Check sheet for the modelled part. Datum: model origin and axes. Units: mm. A direction names the side the tool comes from. Round coordinates to 2 decimals unless told otherwise and drop trailing zeros. Write each loop counter-clockwise with the first axis right and the second up, starting at its lowest first coordinate (ties: lowest second). Pieces come first, ordered by that corner, then holes.
from build123d import *

# Parameters (mm, degrees)
EXTRUDE_180_DEPTH      = 8
EXTRUDE_START          = 8
SKETCH_2_W             = 6
SKETCH_2_H             = 4
EXTRUDE_456_DEPTH      = 36
EXTRUDE_START_2        = 44
EXTRUDE_180_2_DEPTH    = 3
SKETCH_4_R             = 20
SKETCH_4_R_2           = 4
EXTRUDE_691_DEPTH      = 3
EXTRUDE_744_DEPTH      = 3
SKETCH_6_W             = 10
SKETCH_6_H             = 96
EXTRUDE_1_DEPTH        = 3
EXTRUDE_Y_1_DEPTH      = 3
SKETCH_8_W             = 10
SKETCH_8_H             = 96
EXTRUDE_1_2_DEPTH      = 3
EXTRUDE_Y_1_2_DEPTH    = 3
CUT_EXTRUDE_START      = 44
CUT_EXTRUDE_1136_DEPTH = 3
EXTRUDE_1227_DEPTH     = 3
SKETCH_12_R            = 5
EXTRUDE_1296_DEPTH     = 8
SKETCH_13_R            = 1.6
CUT_EXTRUDE_1367_DEPTH = 3
SKETCH_14_R            = 1.6
CUT_EXTRUDE_1428_DEPTH = 8
SKETCH_15_W            = 600
SKETCH_15_H            = 600
CUT_EXTRUDE_1488_DEPTH = 44
F_2MM_START            = 44
F_2MM_DEPTH            = 3
SKETCH_17_R            = 5
EXTRUDE_M3_DEPTH       = 3
SKETCH_18_R            = 5
EXTRUDE_3_DEPTH        = 3
SKETCH_19_R            = 5
EXTRUDE_4_DEPTH        = 3
SKETCH_20_R            = 1.6
CUT_EXTRUDE_M3_DEPTH   = 3
R7P8_75_R              = 7.8
R3P9_R                 = 3.9
F_2MM_45_47_START      = 44
SKETCH_21_W            = 600
SKETCH_21_H            = 600
F_2MM_45_47_DEPTH      = 1
FILLET_1_R             = 1.4
CHAMFER_1_SIZE         = 5
CHAMFER_1_SIZE_2       = 4.246045496
CHAMFER_1_SIZE_3       = 3.817956769
CHAMFER_1_SIZE_4       = 4.370160244
CHAMFER_1_SIZE_5       = 3.876090347
CHAMFER_1_SIZE_6       = 9.033398393


with BuildPart() as part:
    # 草图1 → Extrude 180 (new body)
    with BuildSketch(Plane.XY):
        Polygon((0, -115), (35.536954353, -109.371499374), (70.801069662, -90.621236665), (96.447115314, -62.633489027), (111.081470023, -29.764190187), (115, 0), (111.081470023, 29.764190187), (96.447115314, 62.633489027), (70.801069662, 90.621236665), (35.536954353, 109.371499374), (0, 115), (0, 111), (34.300886376, 105.567273309), (68.338423761, 87.46919365), (93.092433042, 60.454932887), (107.217766718, 28.728914006), (111, 0), (107.217766718, -28.728914006), (93.092433042, -60.454932887), (68.338423761, -87.46919365), (34.300886376, -105.567273309), (0, -111), align=None)
    extrude(amount=EXTRUDE_180_DEPTH)

    # 草图2 → Extrude 456 (add)
    with BuildSketch(Plane.XY.offset(EXTRUDE_START)):
        Polygon((35.584965419, -103.047126287), (37.439067386, -108.753465385), (33.634841321, -109.989533363), (31.780739354, -104.283194265), align=None)
        with Locations((112, 0)):
            Rectangle(SKETCH_2_W, SKETCH_2_H)
        Polygon((31.780739354, 104.283194265), (33.634841321, 109.989533363), (37.439067386, 108.753465385), (35.584965419, 103.047126287), align=None)
    extrude(amount=EXTRUDE_456_DEPTH)

    # 草图3 → Extrude 180 2 (add)
    with BuildSketch(Plane.XY.offset(EXTRUDE_START_2)):
        Polygon((0, -115), (35.536954353, -109.371499374), (70.801069662, -90.621236665), (96.447115314, -62.633489027), (111.081470023, -29.764190187), (115, 0), (111.081470023, 29.764190187), (96.447115314, 62.633489027), (70.801069662, 90.621236665), (35.536954353, 109.371499374), (0, 115), (0, 109), (33.682852387, 103.665160276), (67.10710081, 85.893172143), (91.415091906, 59.365654817), (105.285915066, 28.211275916), (109, 0), (105.285915066, -28.211275916), (91.415091906, -59.365654817), (67.10710081, -85.893172143), (33.682852387, -103.665160276), (0, -109), align=None)
    extrude(amount=EXTRUDE_180_2_DEPTH)



with BuildPart() as body_2:
    # 草图4 → Extrude 691 (new body)
    with BuildSketch(Plane.XY.offset(EXTRUDE_START_2)):
        Circle(SKETCH_4_R)
        Circle(SKETCH_4_R_2, mode=Mode.SUBTRACT)
    extrude(amount=EXTRUDE_691_DEPTH)


with BuildPart() as part_1:
    add(part.part)

    add(body_2.part)  # Extrude 744 merges body 2
    # 草图5 → Extrude 744 (add)
    with BuildSketch(Plane.XY.offset(EXTRUDE_START_2)):
        Polygon((17, -9), (113, -2.5), (113, 2.5), (17, 9), align=None)
    extrude(amount=EXTRUDE_744_DEPTH)

    # 草图6 → Extrude 1 (add)
    with BuildSketch(Plane.XY.offset(EXTRUDE_START_2)):
        with Locations((0, -64)):
            Rectangle(SKETCH_6_W, SKETCH_6_H)
    extrude(amount=EXTRUDE_1_DEPTH)

    # 草图7 → Extrude Y__-1 (add)
    with BuildSketch(Plane.XY.offset(EXTRUDE_START_2)):
        Polygon((60.213265383, 1.279918343), (91.234949037, -66.240061243), (87.165050963, -68.159938757), (54.786734617, -1.279918343), align=None)
    extrude(amount=EXTRUDE_Y_1_DEPTH)

    # 草图8 → Extrude 1 2 (add)
    with BuildSketch(Plane.XY.offset(EXTRUDE_START_2)):
        with Locations((0, 64)):
            Rectangle(SKETCH_8_W, SKETCH_8_H)
    extrude(amount=EXTRUDE_1_2_DEPTH)

    # 草图9 → Extrude Y__1 2 (add)
    with BuildSketch(Plane.XY.offset(EXTRUDE_START_2)):
        Polygon((54.786734617, 1.279918343), (87.165050963, 68.159938757), (91.234949037, 66.240061243), (60.213265383, -1.279918343), align=None)
    extrude(amount=EXTRUDE_Y_1_2_DEPTH)

    # 草图10 → Cut-Extrude 1136 (cut)
    with BuildSketch(Plane.XY.offset(CUT_EXTRUDE_START)):
        Polygon((18, -4.5), (18, 4.5), (80.33, 0), align=None)
    extrude(amount=CUT_EXTRUDE_1136_DEPTH, mode=Mode.SUBTRACT)

    # 草图11 → Extrude 1227 (add)
    with BuildSketch(Plane.XY.offset(EXTRUDE_START_2)):
        Polygon((-5, -107), (5, -107), (5, -116.208077798), (0, -117), (-3, -115), (-5, -112), align=None)
        Polygon((-5, 107), (5, 107), (5, 116.208077798), (0, 117), (-3, 115), (-5, 112), align=None)
    extrude(amount=EXTRUDE_1227_DEPTH)

    # 草图12 → Extrude 1296 (add)
    with BuildSketch(Plane.XY):
        with Locations((0, 112)):
            Circle(SKETCH_12_R)
        with Locations((0, -112)):
            Circle(SKETCH_12_R)
    extrude(amount=EXTRUDE_1296_DEPTH)

    # 草图13 → Cut-Extrude 1367 (cut)
    with BuildSketch(Plane.XY.offset(CUT_EXTRUDE_START)):
        with Locations((0, 112)):
            Circle(SKETCH_13_R)
        with Locations((0, -112)):
            Circle(SKETCH_13_R)
        with Locations((-6.717514421, -6.717514421)):
            Circle(SKETCH_13_R)
        with Locations((-6.717514421, 6.717514421)):
            Circle(SKETCH_13_R)
        with Locations((6.717514421, -6.717514421)):
            Circle(SKETCH_13_R)
        with Locations((6.717514421, 6.717514421)):
            Circle(SKETCH_13_R)
    extrude(amount=CUT_EXTRUDE_1367_DEPTH, mode=Mode.SUBTRACT)

    # 草图14 → Cut-Extrude 1428 (cut)
    with BuildSketch(Plane.XY):
        with Locations((0, 112)):
            Circle(SKETCH_14_R)
        with Locations((0, -112)):
            Circle(SKETCH_14_R)
    extrude(amount=CUT_EXTRUDE_1428_DEPTH, mode=Mode.SUBTRACT)

    # 草图15 → Cut-Extrude 1488 (cut)
    with BuildSketch(Plane.XY):
        Rectangle(SKETCH_15_W, SKETCH_15_H)
    extrude(amount=CUT_EXTRUDE_1488_DEPTH, mode=Mode.SUBTRACT)

    # 草图16 → 外圈径向加厚2mm (add)
    with BuildSketch(Plane.XY.offset(F_2MM_START)):
        Polygon((0, -117), (36.154988342, -111.273612407), (72.032392613, -92.197258172), (98.12445645, -63.722767097), (113.013321676, -30.281828277), (117, 0), (113.013321676, 30.281828277), (98.12445645, 63.722767097), (72.032392613, 92.197258172), (36.154988342, 111.273612407), (0, 117), (0, 114), (35.227937359, 108.420442858), (70.185408187, 89.833225911), (95.608444746, 62.088849992), (110.115544197, 29.505371142), (114, 0), (110.115544197, -29.505371142), (95.608444746, -62.088849992), (70.185408187, -89.833225911), (35.227937359, -108.420442858), (0, -114), align=None)
    extrude(amount=F_2MM_DEPTH)

    # 草图17 → M3铝柱上定位耳 (add)
    with BuildSketch(Plane.XY.offset(EXTRUDE_START_2)):
        with Locations((35.227937359, -108.420442858)):
            Circle(SKETCH_17_R)
    extrude(amount=EXTRUDE_M3_DEPTH)

    # 草图18 → 凸台-拉伸3 (add)
    with BuildSketch(Plane.XY.offset(EXTRUDE_START_2)):
        with Locations((114, 0)):
            Circle(SKETCH_18_R)
    extrude(amount=EXTRUDE_3_DEPTH)

    # 草图19 → 凸台-拉伸4 (add)
    with BuildSketch(Plane.XY.offset(EXTRUDE_START_2)):
        with Locations((35.227937359, 108.420442858)):
            Circle(SKETCH_19_R)
    extrude(amount=EXTRUDE_4_DEPTH)

    # 草图20 → 三处M3上层固定孔 (cut)
    with BuildSketch(Plane.XY.offset(CUT_EXTRUDE_START)):
        with Locations((35.227937359, -108.420442858)):
            Circle(SKETCH_20_R)
        with Locations((114, 0)):
            Circle(SKETCH_20_R)
        with Locations((35.227937359, 108.420442858)):
            Circle(SKETCH_20_R)
    extrude(amount=CUT_EXTRUDE_M3_DEPTH, mode=Mode.SUBTRACT)

    # 外侧梁根部圆角_R7p8_参考75度桨保
    r7p8_75_edges = [part_1.edges().sort_by_distance(p)[0] for p in [
        (5, -19.364916731, 45.5),
        (-5, -19.364916731, 45.5),
        (-5, 19.364916731, 45.5),
        (5, 19.364916731, 45.5),
    ]]
    fillet(r7p8_75_edges, radius=R7P8_75_R)

    # 端耳外缘圆角_R3p9_轮廓内收
    r3p9_edges = [part_1.edges().sort_by_distance(p)[0] for p in [
        (-5, -112, 45.5),
        (-5, 112, 45.5),
        (-3, -115, 45.5),
        (0, -117, 45.5),
        (0, 117, 45.5),
        (-3, 115, 45.5),
    ]]
    fillet(r3p9_edges, radius=R3P9_R)

    # 草图21 → 统一2mm板厚_上层保留45至47 (cut)
    with BuildSketch(Plane.XY.offset(F_2MM_45_47_START)):
        Rectangle(SKETCH_21_W, SKETCH_21_H)
    extrude(amount=F_2MM_45_47_DEPTH, mode=Mode.SUBTRACT)

    # 圆角1
    fillet_1_edges = [part_1.edges().sort_by_distance(p)[0] for p in [
        (18, -4.5, 46),
        (80.33, 0, 46),
        (18, 4.5, 46),
    ]]
    fillet(fillet_1_edges, radius=FILLET_1_R)

    # 倒角1
    # the kernel refuses this chamfer: 9.033398393, 5, 4.370160244, 4.246045496, 3.876090347, 3.817956769 mm, written as the material it adds along each edge
    with BuildSketch(Plane(origin=(108.631931923, -2.795754609, 45), x_dir=(-0.10321619689960815, -0.9946589449140752, 0), z_dir=(0, 0, 1))) as chamfer_1_piece_1:
        Polygon((CHAMFER_1_SIZE * 0.999621916911, -CHAMFER_1_SIZE * 0.0274958766106), (CHAMFER_1_SIZE_2 * 0.17017326961, -CHAMFER_1_SIZE_2 * 0.985414155772), (0, 0), align=None)
    extrude(amount=2)
    with BuildSketch(Plane(origin=(108.631931923, 2.795754609, 47), x_dir=(-0.9995678495067102, 0.02939581998398161, 0), z_dir=(0, 0, -1))) as chamfer_1_piece_2:
        Polygon((CHAMFER_1_SIZE_2 * 0.999270274205, CHAMFER_1_SIZE_2 * 0.0381958005112), (CHAMFER_1_SIZE * 0.159614119931, CHAMFER_1_SIZE * 0.987179483538), (0, 0), align=None)
    extrude(amount=2)
    with BuildSketch(Plane(origin=(89.191460159, -61.792323046, 45), x_dir=(0.6956068650639778, 0.7184226397294735, 0), z_dir=(0, 0, 1))) as chamfer_1_piece_3:
        Polygon((CHAMFER_1_SIZE * 0.999621916911, CHAMFER_1_SIZE * 0.0274958766106), (CHAMFER_1_SIZE_3 * 0.36240953925, CHAMFER_1_SIZE_3 * 0.932018951466), (0, 0), align=None)
    extrude(amount=2)
    with BuildSketch(Plane(origin=(89.191460159, 61.792323046, 47), x_dir=(-0.4601932489228402, -0.8878187729744403, 0), z_dir=(0, 0, -1))) as chamfer_1_piece_4:
        Polygon((CHAMFER_1_SIZE_3 * 0.998870534427, -CHAMFER_1_SIZE_3 * 0.0475147922669), (CHAMFER_1_SIZE * 0.343666607926, -CHAMFER_1_SIZE * 0.939091722143), (0, 0), align=None)
    extrude(amount=2)
    with BuildSketch(Plane(origin=(5, -108.208077798, 47), x_dir=(-0.03603131014618112, 0.9993506615243469, 0), z_dir=(0, 0, -1)), Plane(origin=(5, 108.208077798, 45), x_dir=(-0.0360313101461817, -0.9993506615243467, 0), z_dir=(0, 0, 1))) as chamfer_1_piece_5:
        Polygon((CHAMFER_1_SIZE_4 * 0.999350661636, CHAMFER_1_SIZE_4 * 0.0360313101502), (CHAMFER_1_SIZE * 0.120745181195, CHAMFER_1_SIZE * 0.992683535281), (0, 0), align=None)
    extrude(amount=2)
    with BuildSketch(Plane(origin=(63.490093255, 5.852233269, 45), x_dir=(0.37520935392057214, 0.9269400955458269, 0), z_dir=(0, 0, 1)), Plane(origin=(63.490093255, -5.852233269, 47), x_dir=(0.37520935392056365, -0.9269400955458303, 0), z_dir=(0, 0, -1))) as chamfer_1_piece_6:
        Polygon((CHAMFER_1_SIZE_5 * 0.998939538699, -CHAMFER_1_SIZE_5 * 0.0460412632699), (CHAMFER_1_SIZE * 0.311734042399, -CHAMFER_1_SIZE * 0.950169399007), (0, 0), align=None)
    extrude(amount=2)
    with BuildSketch(Plane(origin=(57.2062873, -6.277699297, 45), x_dir=(-0.9998189901573707, -0.0190259538708392, 0), z_dir=(0, 0, 1)), Plane(origin=(57.2062873, 6.277699297, 47), x_dir=(-0.9998189901573707, 0.019025953870838982, 0), z_dir=(0, 0, -1))) as chamfer_1_piece_7:
        Polygon((CHAMFER_1_SIZE * 0.998820318674, CHAMFER_1_SIZE * 0.0485589436086), (-CHAMFER_1_SIZE_6 * 0.418542922597, CHAMFER_1_SIZE_6 * 0.908197017112), (0, 0), align=None)
    extrude(amount=2)


solid = part_1.part
1. Sectioned sample at C-C, the plane x = 56. Enter the section's corners in (y, z), plus the area to 3 significant figures.
2. Go/stop test with flat-tipped pins: pin 1 (1 mm diameter, centred on x = 54.5, z = 45.5, fed in from -Y); pin 2 (1 mm diameter, centred on y = -60, z = 46, fed in from -X); pin 3 (0.6 mm diameter, centred on y = 82.5, z = 45.5, fed in from +X). Record where each tip stops, or that it passes through.
3. Sectioned sample at A-A, the plane y = 80.5. Enter the section's corners in (x, z).
4. Release check for a two-part mould opening along Y. For faces 3 (the cylindrical face through (-6.166, 20.576, 45.986)), 4 (the flat face through (98.7, -43, 46)), 5 (the cylindrical face through (36.7, -113.2, 46)) record: released by +Y, released by -Y, zero draft, split by the parting line, or undercut.
5. Sectioned sample at B-B, the plane x = 95.5. Enter the section's corners in (y, z).
6. Sectioned sample at D-D, the plane z = 46.3. Give the number of separate pieces and of enclosed holes in the cut face, plus the area to 3 significant figures.
7. Set-up check for faces 1 (the flat face through (55.881, -100.785, 45.986)), 2 (the flat face through (76.61, -75.52, 45.99)): record each of +Z, -Z, +X, -X, +Y, -Y from which the full face is reachable in a straight line by a thin tool's end or side.
8. Scan lines: line 1 along X through (y, z) = (0, 45.7); line 2 along X through (y, z) = (-23, 45.1); line 3 along Y through (x, z) = (54, 46.3). Record each from-to range of solid material in increasing order.
Computed values:
1. outline: (-100.72, 45) - (-91.8, 45) - (-91.8, 47) - (-100.72, 47) - close; (-9.92, 45) - (-1.76, 45) - (-1.76, 47) - (-9.92, 47) - close; (1.76, 45) - (9.92, 45) - (9.92, 47) - (1.76, 47) - close; (91.8, 45) - (100.72, 45) - (100.72, 47) - (91.8, 47) - close
1. area: 68.3 mm2
2. pin 1: stops at y = -101.79
2. pin 2: stops at x = -5
2. pin 3: stops at x = 81.19
3. outline: (-5, 45) - (5, 45) - (5, 47) - (-5, 47) - close; (72.05, 45) - (82.75, 45) - (82.75, 47) - (72.05, 47) - close
4. face 3: released by +Y
4. face 4: undercut
4. face 5: released by -Y
5. outline: (-66.59, 45) - (-50.19, 45) - (-50.19, 47) - (-66.59, 47) - close; (-3.68, 45) - (3.68, 45) - (3.68, 47) - (-3.68, 47) - close; (50.19, 45) - (66.59, 45) - (66.59, 47) - (50.19, 47) - close
6. separate pieces: 1
6. enclosed holes: 15
6. area: 7,400 mm2
7. face 1: +Z, -Z, +X, -Y
7. face 2: +Z, -Z
8. line 1: x = -20 to -4, 4 to 18, 62.29 to 112.4, 115.6 to 119
8. line 2: x = -5.18 to 5.18, 65.3 to 71.37, 105.97 to 113.97
8. line 3: y = -101.79 to -92.86, -8.17 to -1.9, 1.9 to 8.17, 92.86 to 101.79
